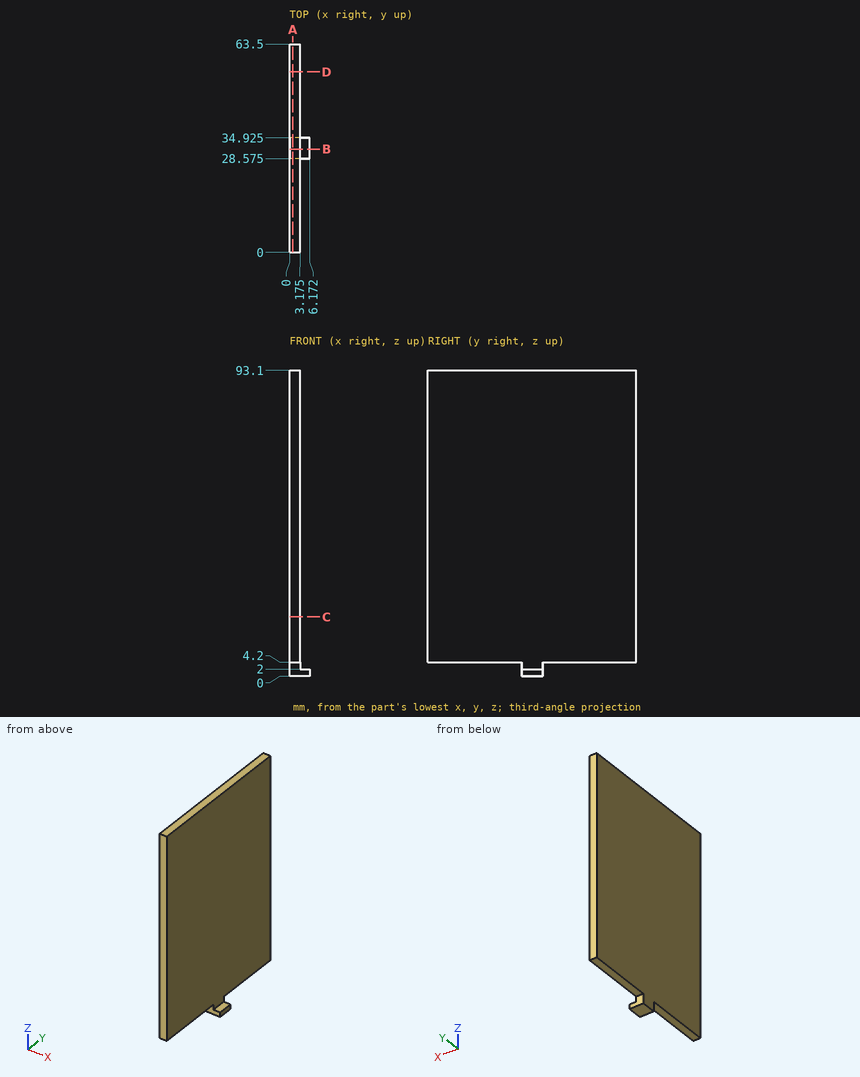
Check sheet for the drawn part. Datum: minimum x, y, z corner. Units: mm. Round coordinates to 2 decimals unless told otherwise and drop trailing zeros. Order: outer loops, then holes, each group sorted by start corner. A loop starts at its lowest first (then second) coordinate and runs counter-clockwise, first axis right, second up. Notation, with made-up numbers: (1.5, 1) -> (24.5, 1) arc R23 cw to (24.5, 21) -> close; hole circle Ø7 at (31, -8.5). An arc over 180 degrees is marked (long way). Put each result on its own line as item: value. Start each with the question number.
(1) Section check B-B (y = 31.5). Enter the section's corners in (x, z) (1 decimal).
(2) Depth check by flat-ended pin: pin 1 Ø10 at (y, z) = (31, 36) entering from +X (3 decimals); pin 2 Ø1 at (x, y) = (1, 50.5) entering from -Z; pin 3 Ø3.5 at (x, y) = (5, 33) entering from +Z. Enter the tip coordinate at first touch or a pass-through.
(3) Material ranges on line 1 along X through (y, z) = (58, 67.5) (3 decimals); line 2 along Z through (x, y) = (1.25, 36), recorded low to high.
(4) Section check D-D (y = 55). Enter the section's corners in (x, z) (3 decimals).
(5) Section check C-C (z = 18). Enter the section's corners in (x, y) (3 decimals).
(6) Section check A-A (x = 1). Enter the section's corners in (y, z) (3 decimals), then the cut area to 3 significant figures.
Completed:
1. outline: (0, 0) -> (6.2, 0) -> (6.2, 2) -> (3.2, 2) -> (3.2, 93.1) -> (0, 93.1) -> close
2. pin 1: stops at x = 3.175
2. pin 2: stops at z = 4.2
2. pin 3: stops at z = 2
3. line 1: x = 0 to 3.175
3. line 2: z = 4.2 to 93.1
4. outline: (0, 4.2) -> (3.175, 4.2) -> (3.175, 93.1) -> (0, 93.1) -> close
5. outline: (0, 0) -> (3.175, 0) -> (3.175, 63.5) -> (0, 63.5) -> close
6. outline: (0, 4.2) -> (28.575, 4.2) -> (28.575, 0) -> (34.925, 0) -> (34.925, 4.2) -> (63.5, 4.2) -> (63.5, 93.1) -> (0, 93.1) -> close
6. area: 5,670 mm2
